```python
from build123d import *

# Parameters (mm, degrees)
F0_W     = 300
F0_H     = 400
F1_DEPTH = 19
F3_DEPTH = 8
F4_W     = 30
F4_H     = 30
F5_DEPTH = 11


with BuildPart() as f1:
    # F0 (on Front) → F1 (new body)
    with BuildSketch(Plane.XZ):
        with Locations((-14.034653, 10.167784)):
            Rectangle(F0_W, F0_H)
    extrude(amount=F1_DEPTH)

    # F2 (on face) → F3 (cut)
    with BuildSketch(Plane(origin=(0, 0, 0), x_dir=(-1, 0, 0), z_dir=(0, 1, 0))):
        Polygon((-125.465347, 200.167784), (-125.465347, -167.832216), (-95.465347, -167.832216), (-95.465347, 170.167784), (-83.965347, 170.167784), (-83.965347, -167.832216), (-12.465347, -167.832216), (-12.465347, 170.167784), (-0.965347, 170.167784), (-0.965347, -167.832216), (70.534653, -167.832216), (70.534653, 170.167784), (82.034653, 170.167784), (82.034653, -167.832216), (153.534653, -167.832216), (153.534653, 200.167784), (123.534653, 200.167784), (123.534653, -137.832216), (112.034653, -137.832216), (112.034653, 200.167784), (40.534653, 200.167784), (40.534653, -137.832216), (29.034653, -137.832216), (29.034653, 200.167784), (-42.465347, 200.167784), (-42.465347, -137.832216), (-53.965347, -137.832216), (-53.965347, 200.167784), align=None)
    extrude(amount=-F3_DEPTH, mode=Mode.SUBTRACT)

    # F4 (on face) → F5 (cut)
    with BuildSketch(Plane(origin=(0, -8, 0), x_dir=(-1, 0, 0), z_dir=(0, 1, 0))):
        with Locations((138.534653, 185.167784)):
            Rectangle(F4_W, F4_H)
    extrude(amount=-F5_DEPTH, mode=Mode.SUBTRACT)


solid = f1.part
```
Here's how the part is built. I have some questions about the finished solid (model axes, mm). A direction names the side the tool comes from. Coordinates: 2 decimals unless noted, no trailing zeros. Write each loop counter-clockwise with the first axis right and the second up, starting at its lowest first coordinate (ties: lowest second). Pieces come first, ordered by that corner, then holes. Notation, with made-up numbers: (-31, -7) - (1, -7) arc R14 ccw to (1, 11) - close; hole circle Ø6 at (77, 25.25). An arc over 180 degrees is marked (long way). One line per item, written item: value.
1) Suppose I cut it at D-D on x = -76.5. Write out the boundary of the cut face in (y, z), and give its area (3 significant figures).
Model answer:
outline: (-19, -189.83) - (0, -189.83) - (0, 170.17) - (-8, 170.17) - (-8, 200.17) - (0, 200.17) - (0, 210.17) - (-19, 210.17) - close
area: 7,360 mm²
2) I need wall thicknesses on line 1 along Z through (x, y) = (-118.5, -4.5); line 2 along Z through (x, y) = (79, -3); line 3 along Y through (x, z) = (-42.5, -158). Which ranges of each line are inside material? Lowest first, please.
Model answer:
line 1: z = -189.83 to -167.83, -137.83 to 210.17
line 2: z = -189.83 to -167.83, 200.17 to 210.17
line 3: y = -19 to -8
3) On a 3-axis mill with a long thin cutter (end or side, diameter ignored), from which of +Z, -Z, +X, -X, +Y, -Y can I reach the whole of each face in a straight line? I mean faces 3 (the flat face through (-138, -13, 170.168)), 4 (the flat face through (95.465, -4, -1)). Say none if no direction works.
Model answer:
face 3: +Y, -Y
face 4: +Y
4) Suppose I cut it at A-A on x = -141.5. Write out the boundary of the cut face in (y, z).
Model answer:
outline: (-19, -189.83) - (0, -189.83) - (0, -167.83) - (-8, -167.83) - (-8, 170.17) - (-19, 170.17) - close; (-19, 200.17) - (0, 200.17) - (0, 210.17) - (-19, 210.17) - close
5) We'd pull the mould along X, two halves only. Please class faces 1 (the flat face through (135.965, -9, 7)), 2 (the flat face through (-34, -4, -167.832)): pulls with the +X half, pulls with the -X half, needs draft (parallel to the pull), parting line crosses it, or undercut.
Model answer:
face 1: pulls with the +X half
face 2: undercut
